```python
from build123d import *

# Parameters (mm, degrees)
CROQUIS1_R              = 2.5
SALIENTE_EXTRUIR1_DEPTH = 5
CORTAR_EXTRUIR1_START   = -10
CORTAR_EXTRUIR1_DEPTH   = 10
CORTAR_EXTRUIR2_DEPTH   = 10


with BuildPart() as part:
    # Croquis1 → Saliente-Extruir1 (new body)
    with BuildSketch(Plane(origin=(0, 0, 0), x_dir=(1, 0, 0), z_dir=(0, 1, 0))):
        with BuildLine():
            Line((-6, 7.413947971), (-6, 3.413947971))
            Line((-6, 3.413947971), (-3.653075314, 3.413947971))
            ThreePointArc((-3.653075314, 3.413947971), (0, -5), (3.653075314, 3.413947971))
            Line((3.653075314, 3.413947971), (6, 3.413947971))
            Line((6, 3.413947971), (6, 7.413947971))
            ThreePointArc((6, 7.413947971), (0, 5), (-6, 7.413947971))
        make_face()
        with Locations(Location((0, 0, 0), (0, 0, 270))):
            Circle(CROQUIS1_R, mode=Mode.SUBTRACT)
    extrude(amount=SALIENTE_EXTRUIR1_DEPTH)

    # Croquis2 → Cortar-Extruir1 (cut)
    with BuildSketch(Plane(origin=(0, 5, 0), x_dir=(1, 0, 0), z_dir=(0, 1, 0)).offset(CORTAR_EXTRUIR1_START)):
        with BuildLine():
            ThreePointArc((2.4311737, -0.582575695), (1.548153862, -1.96296195), (0, -2.5))
            Line((0, -2.5), (0, -5))
            ThreePointArc((0, -5), (1.021548218, -4.894531565), (2, -4.582575695))
            Line((2, -4.582575695), (2.4311737, -0.582575695))
        make_face()
        with BuildLine():
            Line((0, -5), (0, -2.5))
            ThreePointArc((0, -2.5), (-1.548153862, -1.96296195), (-2.4311737, -0.582575695))
            Line((-2.4311737, -0.582575695), (-2, -4.582575695))
            ThreePointArc((-2, -4.582575695), (-1.021548218, -4.894531565), (0, -5))
        make_face()
    extrude(amount=CORTAR_EXTRUIR1_DEPTH, mode=Mode.SUBTRACT)

    # Croquis3 → Cortar-Extruir2 (cut)
    with BuildSketch(Plane(origin=(0, 5, 0), x_dir=(1, 0, 0), z_dir=(0, 1, 0))):
        Polygon((3.653075314, 3.413947971), (6, 5.413947971), (6, 3.413947971), align=None)
        Polygon((-3.653075314, 3.413947971), (-6, 5.413947971), (-6, 3.413947971), align=None)
    extrude(amount=-CORTAR_EXTRUIR2_DEPTH, mode=Mode.SUBTRACT)


solid = part.part
```
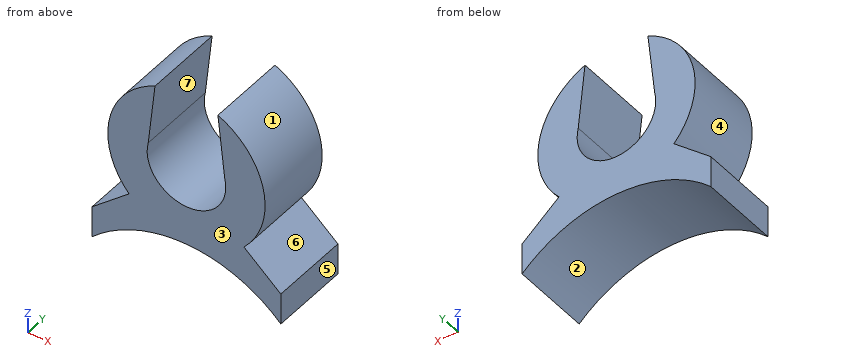
Verification items for the finished model (mm, model axes). Face numbers are marked on the shaded views. A direction names the side the tool comes from. Coordinates: 2 decimals unless noted, no trailing zeros. Loops run counter-clockwise (first coordinate to the right, second up) from the corner with the lowest first, then second, coordinate; pieces in that order, holes last. Notation, with made-up numbers: (54.25, -32.75) - (72.25, -32.75) arc R33 cw to (72.25, 4.25) - close; hole circle Ø2 at (-1.5, -13.75). An arc over 180 degrees is marked (long way). Return JSON: item names as keys, results as strings.
1. Thickness scan on L1, parallel to X at y = 3.35, z = 0; L2, parallel to X at y = 3.8, z = 1; L3, parallel to Z at x = -4, y = 4.1. Record the ranges inside material, lowest first.
Established:
{"L1": "x = -5 to -2.5, 2.5 to 5", "L2": "x = -4.9 to -2.39, 2.39 to 4.9", "L3": "z = -5.98 to -3.71, -3 to 3"}
2. Mould release check, pull along Z, two halves, no side actions. Record for the marked faces 1, 2, 3 and 4: +Z half, -Z half, draft (parallel to the pull), parting line (faces both ways), or undercut.
Established:
{"face 1": "undercut", "face 2": "-Z half", "face 3": "draft", "face 4": "undercut"}
3. Section check A-A, the plane z = 0. Record the boundary of the cut face in (x, y), then the cut area to 3 significant figures.
Established:
{"outline": "(-5, 0) - (-2.5, 0) - (-2.5, 5) - (-5, 5) - close; (2.5, 0) - (5, 0) - (5, 5) - (2.5, 5) - close", "area": "25.0 mm2"}
4. Go/stop test with a flat-tipped pin: pin 1 (3 mm diameter, centred on y = 2.5, z = 0, fed in from +X). Record where the tip stops, or that it passes through.
Established:
{"pin 1": "stops at x = 5"}
5. Section check D-D, the plane x = 0. Record the boundary of the cut face in (y, z), then the cut area to 3 significant figures.
Established:
{"outline": "(0, -5) - (5, -5) - (5, -2.5) - (0, -2.5) - close", "area": "12.5 mm2"}
6. Tool access check on the marked faces 5, 6 and 7. Record the directions out of +Z, -Z, +X, -X, +Y, -Y that give a thin tool (end or side, any length) a straight path to the whole face; none if there is none.
Established:
{"face 5": "+Z, -Z, +X, +Y, -Y", "face 6": "+X, +Y, -Y", "face 7": "+Y, -Y"}
7. Section check B-B, the plane x = -4.5. Record the boundary of the cut face in (y, z), then the cut area to 3 significant figures.
Established:
{"outline": "(0, -6.26) - (5, -6.26) - (5, -4.14) - (0, -4.14) - close; (0, -2.18) - (5, -2.18) - (5, 2.18) - (0, 2.18) - close", "area": "32.4 mm2"}
8. Section check C-C, the plane y = 3.7. Record the boundary of the cut face in (x, z).
Established:
{"outline": "(-6, -7.41) arc R8.66 cw to (6, -7.41) - (6, -5.41) - (3.65, -3.41) arc R5 ccw to (2, 4.58) - (2.43, 0.58) arc R2.5 cw (long way) to (-2.43, 0.58) - (-2, 4.58) arc R5 ccw to (-3.65, -3.41) - (-6, -5.41) - close"}
